Read the model definition and answer for the solid it produces. Units are mm, in the model's axes. A direction names the side the tool comes from. Give positions to 0.01 mm unless a question says otherwise; leave off trailing zeros. Loops run counter-clockwise (first coordinate to the right, second up) from the corner with the lowest first, then second, coordinate; pieces in that order, holes last. Notation, with made-up numbers: (88, -29.5) - (143, -29.5) arc R37 cw to (143, 9.5) - close; hole circle Ø7 at (14.25, 24.5). An arc over 180 degrees is marked (long way). Use a Markdown table: item, result. Add a question column.
Item 1: For a pull along Z with two mould halves and no side action, classify faces 5 (the face through (-90.77, 2, 12)), 6 (the face through (55.28, 70, 68)), 7 (the face through (-22, 38, 69.527)) as +Z half, -Z half, draft (parallel to the pull), parting line (faces both ways), or undercut.
Item 2: Consider probe 1 along Z at (x, y) = (-70, 32); probe 2 along Y at (x, z) = (17, 50.5) (3 decimals); probe 3 along X at (y, z) = (63, 68). Determine where each line is inside the solid, lowest interval first. Write a range as [from, to].
Item 3: This flat-tipped pin is pushed along its axis until it touches: P1, Ø2.5, axis at y = 1, z = 14.5, coming from the +X side. Where does it stop, or does it pass through?
Item 4: A cutting plane is placed at B-B (x = 42.5). Determine the outline of the cut face in (y, z).
Item 5: Which of the six approach directions +Z, -Z, +X, -X, +Y, -Y give full straight-line access (tool end or side, diameter ignored) to faces 1 (the face through (-41, 73.025, 12)), 2 (the face through (-10.898, 1.565, 11.644)), 3 (the face through (17.18, 2, 13)), 4 (the face through (43.886, 32.194, 67.917))?
Item 6: A cutting plane is placed at D-D (x = -36). Determine the outline of the cut face in (y, z) (3 decimals), plus the area to 3 significant figures.
Item 7: A cutting plane is placed at C-C (y = 16.5). Determine the outline of the cut face in (x, z), plus the area to 3 significant figures.
Item 8: A cutting plane is placed at A-A (z = 6). Determine the outline of the cut face in (x, y) (1 decimal), plus the area to 3 significant figures.
from build123d import *

# Parameters (mm, degrees)
SKETCH1_W               = 152.4
SKETCH1_H               = 114.3
BOSS_EXTRUDE1_DEPTH     = 76.2
CUT_EXTRUDE1_DEPTH      = 142.677746119
CUT_EXTRUDE1_DEPTH_BACK = 142.677746119
SKETCH5_W               = 38.1
SKETCH5_H               = 107.95
CUT_EXTRUDE4_DEPTH      = 142.677746119
CUT_EXTRUDE5_DEPTH      = 169.235334824
CUT_EXTRUDE5_DEPTH_BACK = 169.235334824
SKETCH6_R               = 7.9375
SKETCH8_W               = 107.95
SKETCH8_H               = 69.85
CUT_EXTRUDE6_DEPTH      = 185.027568212
SKETCH9_R               = 1.5875
CUT_EXTRUDE7_DEPTH      = 3.175
SKETCH10_W              = 63.5
SKETCH10_H              = 19.05
CUT_EXTRUDE8_DEPTH      = 5.715


with BuildPart() as part:
    # Sketch1 → Boss-Extrude1 (new body)
    with BuildSketch(Plane(origin=(0, 0, 0), x_dir=(1, 0, 0), z_dir=(0, 1, 0))):
        with Locations((-20.919503106, -12.376583851)):
            Rectangle(SKETCH1_W, SKETCH1_H)
    extrude(amount=BOSS_EXTRUDE1_DEPTH)

    # Sketch3 → Cut-Extrude1 (cut, two sides: drawn at the far end of the back side and taken through both)
    with BuildSketch(Plane.XY.offset(-CUT_EXTRUDE1_DEPTH_BACK)):
        Polygon((55.280496894, 63.5), (32.168387019, 0), (55.280496894, 0), align=None)
    extrude(amount=CUT_EXTRUDE1_DEPTH + CUT_EXTRUDE1_DEPTH_BACK, mode=Mode.SUBTRACT)

    # Sketch5 → Cut-Extrude4 (cut, through all)
    with BuildSketch(Plane(origin=(0, 0, 0), x_dir=(1, 0, 0), z_dir=(0, 1, 0))):
        with Locations((36.230496894, -12.376583851)):
            Rectangle(SKETCH5_W, SKETCH5_H)
    extrude(amount=CUT_EXTRUDE4_DEPTH, mode=Mode.SUBTRACT)

    # Sketch6 → Cut-Extrude5 (cut, two sides: drawn at the far end of the back side and taken through both)
    with BuildSketch(Plane.XY.offset(69.526583851).offset(-CUT_EXTRUDE5_DEPTH_BACK)):
        with Locations((39.405496894, 63.5)):
            Circle(SKETCH6_R)
    extrude(amount=CUT_EXTRUDE5_DEPTH + CUT_EXTRUDE5_DEPTH_BACK, mode=Mode.SUBTRACT)

    # Sketch8 → Cut-Extrude6 (cut, through all)
    with BuildSketch(Plane.ZY.offset(97.119503106)):
        with Locations((12.376583851, 38.1)):
            Rectangle(SKETCH8_W, SKETCH8_H)
    extrude(amount=-CUT_EXTRUDE6_DEPTH, mode=Mode.SUBTRACT)

    # Sketch9 → Cut-Extrude7 (cut)
    with BuildSketch(Plane.XZ):
        with Locations(Location((4.480496894, 12.376583851, 0), (0, 0, 270))):
            Circle(SKETCH9_R)
        with Locations(Location((-9.489503106, 12.376583851, 0), (0, 0, 270))):
            Circle(SKETCH9_R)
    extrude(amount=-CUT_EXTRUDE7_DEPTH, mode=Mode.SUBTRACT)

    # Sketch10 → Cut-Extrude8 (cut)
    with BuildSketch(Plane.XZ):
        with Locations((-59.019503106, 12.376583851)):
            Rectangle(SKETCH10_W, SKETCH10_H)
    extrude(amount=-CUT_EXTRUDE8_DEPTH, mode=Mode.SUBTRACT)


solid = part.part
Geometry says:
| question | item | result |
|---|---|---|
| 1 | face 5 | undercut |
| 1 | face 6 | draft |
| 1 | face 7 | +Z half |
| 2 | probe 1 | [-44.77, -41.6], [66.35, 69.53] |
| 2 | probe 2 | [0, 3.175], [73.025, 76.2] |
| 2 | probe 3 | [-97.12, 31.48], [47.33, 55.1] |
| 3 | P1 | x = 17.18 |
| 4 | outline | (28.39, -44.77) - (56.19, -44.77) - (56.19, -41.6) - (28.39, -41.6) - close; (28.39, 66.35) - (56.19, 66.35) - (56.19, 69.53) - (28.39, 69.53) - close; (70.81, -44.77) - (76.2, -44.77) - (76.2, -41.6) - (70.81, -41.6) - close; (70.81, 66.35) - (76.2, 66.35) - (76.2, 69.53) - (70.81, 69.53) - close |
| 5 | face 1 | +X, -X |
| 5 | face 2 | -Y |
| 5 | face 3 | +X, +Y, -Y |
| 5 | face 4 | +Z, -Z, +X, -Y |
| 6 | outline | (0, -44.773) - (76.2, -44.773) - (76.2, 69.527) - (0, 69.527) - (0, 21.902) - (3.175, 21.902) - (3.175, 66.352) - (73.025, 66.352) - (73.025, -41.598) - (3.175, -41.598) - (3.175, 2.852) - (0, 2.852) - close |
| 6 | area | 1,110 mm² |
| 7 | outline | (-97.12, -44.77) - (38.17, -44.77) - (38.17, -41.6) - (-97.12, -41.6) - close; (-97.12, 66.35) - (38.17, 66.35) - (38.17, 69.53) - (-97.12, 69.53) - close |
| 7 | area | 859 mm² |
| 8 | outline | (-97.1, 0) - (-90.8, 0) - (-90.8, 3.2) - (-97.1, 3.2) - close; (-97.1, 73) - (17.2, 73) - (17.2, 76.2) - (-97.1, 76.2) - close; (-27.3, 0) - (17.2, 0) - (17.2, 3.2) - (-27.3, 3.2) - close |
| 8 | area | 524 mm² |
